Input: part model. Units: mm. Frame: model coordinates. Coordinates: 2 decimals unless noted, no trailing zeros. Loops run counter-clockwise (first coordinate to the right, second up) from the corner with the lowest first, then second, coordinate; pieces in that order, holes last.
Item 1: Section A-A on y = -5. Return loops of the section in (x, z).
Item 2: Contact query for a flat-ended pin moving along its axis: P1, Ø2, axis at x = 228.5, y = -2.5, coming from the +Z side. Output: stop coordinate, or through.
Item 3: Section B-B on x = 172.5. Return loops of the section in (y, z), and give its area (3 significant figures).
Item 4: Ray query, line 1 along Z through (x, y) = (185.5, -2.5); line 2 along Z through (x, y) = (247.5, -2.75); line 3 along X through (y, z) = (-3.75, -33.5). Return the intervals inside material, ascending.
Item 5: Section C-C on z = -25.5. Return loops of the section in (x, y), and give its area (3 significant figures).
```python
from build123d import *

# Parameters (mm, degrees)
F1_DEPTH    = 6
F2_T1_DEPTH = 31.7168298797
F2_T3_DEPTH = 26.6288680093


# Not quite as in the source:
# - a fillet or chamfer that OpenCascade refuses, or shapes differently, is made with other operations: its cross-section is extruded or revolved along the edge and cut away or added


with BuildPart() as f1:
    # F0 (on Front) → F1 (new body)
    with BuildSketch(Plane.XZ):
        Polygon((202.5005221367, 0), (155.6514501572, -47.4510490894), (271.2386846542, -93.6057344079), (281.0647502264, -77.5675406007), align=None)
    extrude(amount=F1_DEPTH)

    # F2: chamfer of 5 on 2 edges, made by hand

    # F2_s2 → F2_t1 (cut)
    with BuildSketch(Plane.XZ.offset(-12.8584149398)):
        Polygon((198.9876293479, -3.5580309518), (206.0585530885, -3.5128927888), (202.5005221367, 0), align=None)
    extrude(amount=F2_T1_DEPTH, mode=Mode.SUBTRACT)

    # F2_s4 → F2_t3 (cut)
    with BuildSketch(Plane.XZ.offset(-10.3144340046)):
        Polygon((278.9922098799, -80.9503598488), (278.2416469809, -74.7802520225), (281.0647502264, -77.5675406007), align=None)
    extrude(amount=F2_T3_DEPTH, mode=Mode.SUBTRACT)


solid = f1.part
```
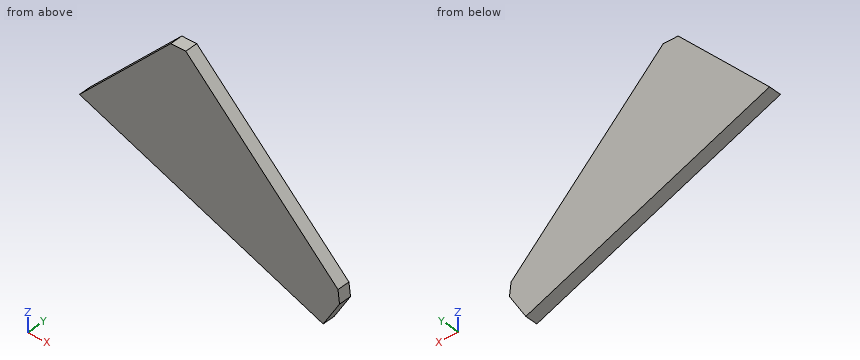
Results found:
1. outline: (155.65, -47.45) - (271.24, -93.61) - (278.99, -80.95) - (278.24, -74.78) - (206.06, -3.51) - (198.99, -3.56) - close
2. P1: stops at z = -24.68
3. outline: (-6, -54.18) - (0, -54.18) - (0, -30.39) - (-6, -30.39) - close
3. area: 143 mm2
4. line 1: z = -59.37 to -17.22
4. line 2: z = -84.13 to -44.43
4. line 3: x = 169.43 to 236.43
5. outline: (177.32, -6) - (228.33, -6) - (228.33, 0) - (177.32, 0) - close
5. area: 306 mm2
